Geometry check sheet. Reference: drawing and pictorial views, mm from the part's lowest x, y, z. A direction names the side the tool comes from. Round coordinates to 2 decimals unless told otherwise and drop trailing zeros. Loops run counter-clockwise (first coordinate to the right, second up) from the corner with the lowest first, then second, coordinate; pieces in that order, holes last. Notation, with made-up numbers: (80.5, 89.5) -> (122.5, 89.5) arc R23 ccw to (122.5, 102.5) -> close; hole circle Ø6 at (35, -13). An arc over 180 degrees is marked (long way). Use one line per item in the form item = value.
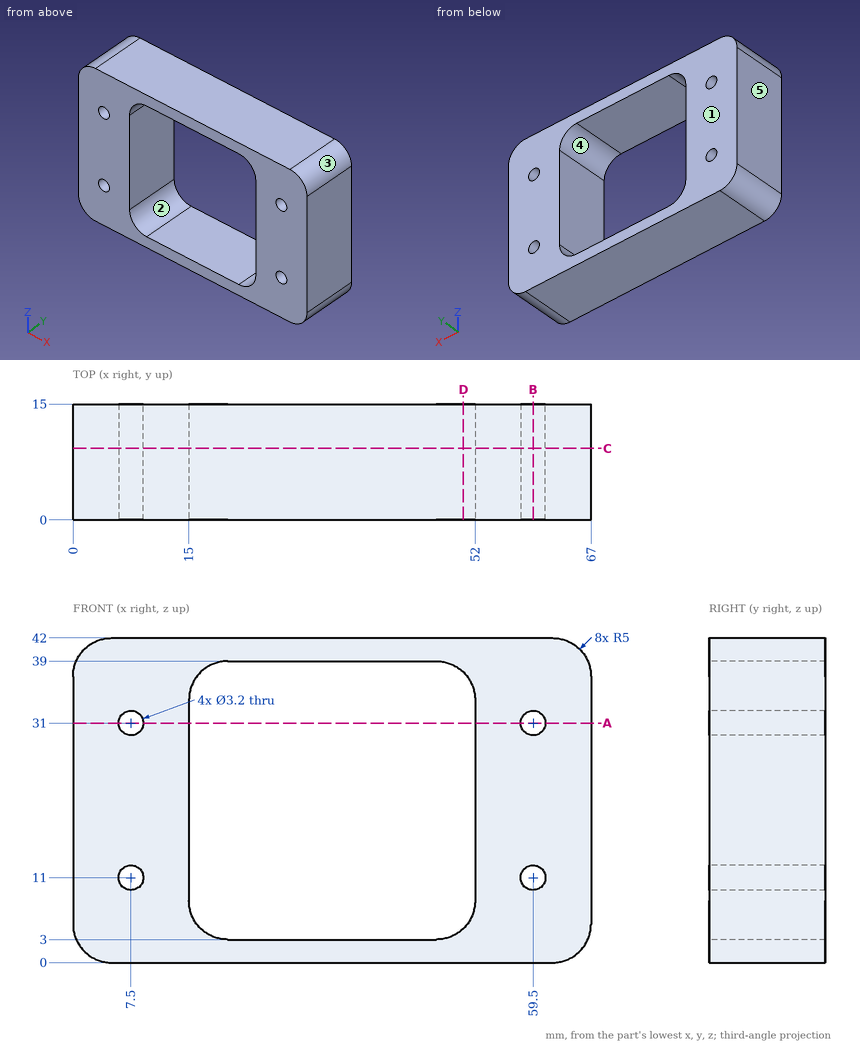
1. Mould release check, pull along X, two halves, no side actions. Record for the marked faces 3, 4 and 5: released by +X, released by -X, zero draft, split by the parting line, or undercut.
Return value:
face_3 = released by +X
face_4 = undercut
face_5 = released by -X
2. Section check C-C (y = 9.25). Record the boundary of the cut face in (x, z).
Return value:
outline = (0, 5) arc R5 ccw to (5, 0) -> (62, 0) arc R5 ccw to (67, 5) -> (67, 37) arc R5 ccw to (62, 42) -> (5, 42) arc R5 ccw to (0, 37) -> close; hole circle Ø3.2 at (7.5, 11); hole circle Ø3.2 at (7.5, 31); hole (15, 8) arc R5 ccw to (20, 3) -> (47, 3) arc R5 ccw to (52, 8) -> (52, 34) arc R5 ccw to (47, 39) -> (20, 39) arc R5 ccw to (15, 34) -> close; hole circle Ø3.2 at (59.5, 11); hole circle Ø3.2 at (59.5, 31)
3. Gauge pin test, flat ends, axial feed: pin 1 (12 mm diameter, centred on x = 32, z = 11.5, fed in from -Y); pin 2 (5 mm diameter, centred on x = 59.5, z = 31, fed in from +Y). Record the tip position at first contact, or that the pin passes through.
Return value:
pin_1 = through
pin_2 = 15
4. Tool access check on the marked faces 1 and 2. Record the directions out of +Z, -Z, +X, -X, +Y, -Y that give a thin tool (end or side, any length) a straight path to the whole face; none if there is none.
Return value:
face_1 = +Z, -Z, +X, -X, +Y
face_2 = +Y, -Y
5. Material ranges on line 1 along X through (y, z) = (6.5, 11); line 2 along Z through (x, y) = (59.5, 7.75); line 3 along X through (y, z) = (12, 22.5), recorded low to high.
Return value:
line_1 = 0 to 5.9, 9.1 to 15, 52 to 57.9, 61.1 to 67
line_2 = 0 to 9.4, 12.6 to 29.4, 32.6 to 42
line_3 = 0 to 15, 52 to 67
6. Section check A-A (z = 31). Record the boundary of the cut face in (x, y), then the cut area to 3 significant figures.
Return value:
outline = (0, 0) -> (5.9, 0) -> (5.9, 15) -> (0, 15) -> close; (9.1, 0) -> (15, 0) -> (15, 15) -> (9.1, 15) -> close; (52, 0) -> (57.9, 0) -> (57.9, 15) -> (52, 15) -> close; (61.1, 0) -> (67, 0) -> (67, 15) -> (61.1, 15) -> close
area = 354 mm2
7. Section check B-B (x = 59.5). Record the boundary of the cut face in (y, z).
Return value:
outline = (0, 0) -> (15, 0) -> (15, 9.4) -> (0, 9.4) -> close; (0, 12.6) -> (15, 12.6) -> (15, 29.4) -> (0, 29.4) -> close; (0, 32.6) -> (15, 32.6) -> (15, 42) -> (0, 42) -> close
8. Section check D-D (x = 50.5). Record the boundary of the cut face in (y, z).
Return value:
outline = (0, 0) -> (15, 0) -> (15, 4.43) -> (0, 4.43) -> close; (0, 37.57) -> (15, 37.57) -> (15, 42) -> (0, 42) -> close
